Answer from the drawing. Dimensions are ordinates in mm from the lowest x, y and z of the part. A direction names the side the tool comes from. Coordinates: 2 decimals unless noted, no trailing zeros. Write each loop counter-clockwise with the first axis right and the second up, starting at its lowest first coordinate (ties: lowest second). Pieces come first, ordered by that corner, then holes. Notation, with made-up numbers: (-19, -21) - (28, -21) arc R20 cw to (28, -13) - close; hole circle Ø2 at (1.5, 41.5). An arc over 180 degrees is marked (long way). Return JSON: item names as keys, results as strings.
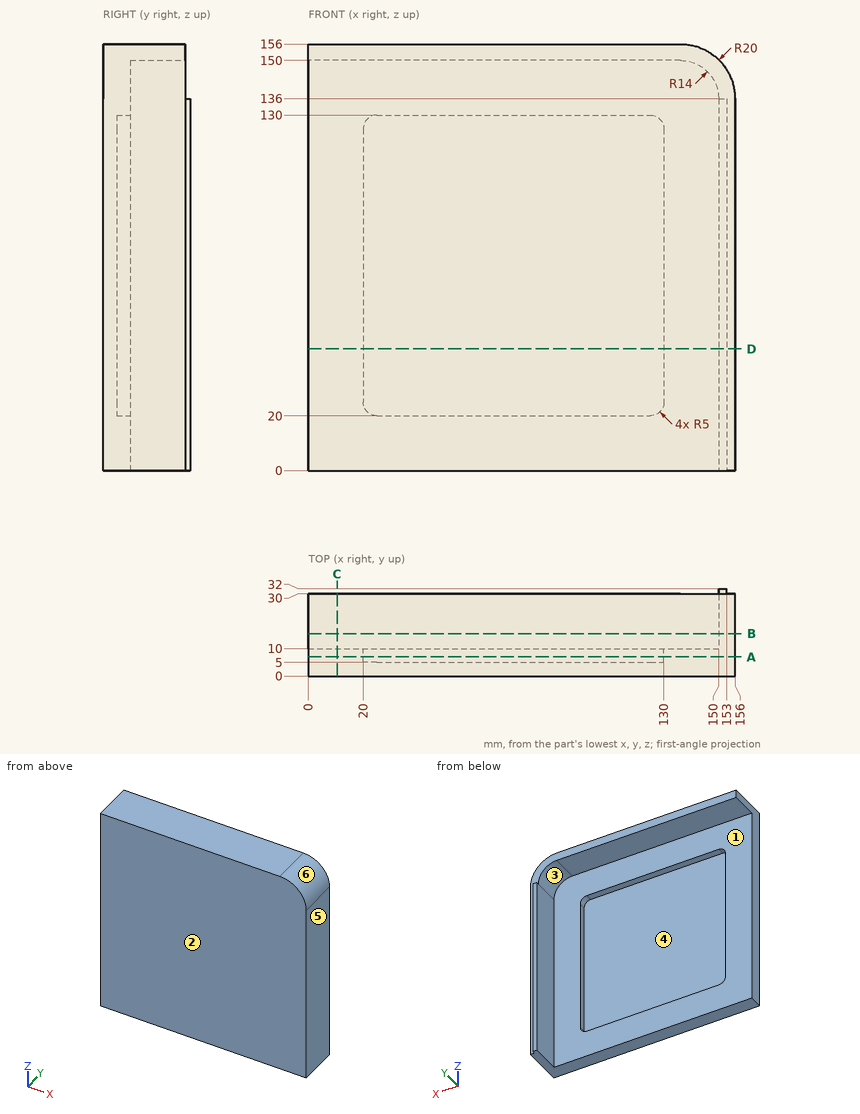
(1) Flat-ended cylindrical pins translate along their axes: P1, Ø1.5, axis at x = 88, z = 89, coming from the +Y side; P2, Ø0.6, axis at x = 151.5, y = 30.5, coming from the +Z side; P3, Ø12, axis at x = 22, y = 18.5, coming from the -Z side. Find the tip coordinate at first contact, or state that the pin passes through.
Answer:
{"P1": "y = 5", "P2": "z = 136", "P3": "z = 150"}
(2) A cutting plane is placed at A-A (y = 7). Determine the outline of the cut face in (x, z), and give its area (3 significant figures).
Answer:
{"outline": "(0, 0) - (156, 0) - (156, 136) arc R20 ccw to (136, 156) - (0, 156) - close; hole (20, 25) arc R5 ccw to (25, 20) - (125, 20) arc R5 ccw to (130, 25) - (130, 125) arc R5 ccw to (125, 130) - (25, 130) arc R5 ccw to (20, 125) - close", "area": "12,200 mm²"}
(3) A cutting plane is placed at B-B (y = 15.5). Determine the outline of the cut face in (x, z).
Answer:
{"outline": "(0, 150) - (136, 150) arc R14 cw to (150, 136) - (150, 0) - (156, 0) - (156, 136) arc R20 ccw to (136, 156) - (0, 156) - close"}
(4) Which of the six approach directions +Z, -Z, +X, -X, +Y, -Y give full straight-line access (tool end or side, diameter ignored) to the marked faces 1 and 2?
Answer:
{"face 1": "-Z, -X, +Y", "face 2": "+Z, -Z, +X, -X, -Y"}
(5) Straight lines are drawn through the part: line 1 (Z direction, x = 32, y = 8.5); line 2 (Z direction, x = 123, y = 11). For each, find the intervals that lie inside material, in ascending order. Write a range as from..to.
Answer:
{"line 1": "0..20, 130..156", "line 2": "150..156"}
(6) A cutting plane is placed at D-D (z = 44.5). Determine the outline of the cut face in (x, y).
Answer:
{"outline": "(0, 0) - (156, 0) - (156, 30) - (153, 30) - (153, 32) - (150, 32) - (150, 10) - (130, 10) - (130, 5) - (20, 5) - (20, 10) - (0, 10) - close"}
(7) Determine the mould class of the marked faces 3, 4, 5 and 6 for opening direction Z: +Z half, -Z half, draft (parallel to the pull), parting line (faces both ways), or undercut.
Answer:
{"face 3": "-Z half", "face 4": "undercut", "face 5": "draft", "face 6": "+Z half"}
(8) A cutting plane is placed at C-C (x = 10.5). Determine the outline of the cut face in (y, z).
Answer:
{"outline": "(0, 0) - (10, 0) - (10, 150) - (30, 150) - (30, 156) - (0, 156) - close"}
